Part model, mm, in its own coordinate system. Face numbers are marked on the shaded views. A direction names the side the tool comes from. Coordinates: 2 decimals unless noted, no trailing zeros. Write each loop counter-clockwise with the first axis right and the second up, starting at its lowest first coordinate (ties: lowest second). Pieces come first, ordered by that corner, then holes. Notation, with made-up numbers: (-2, -15.5) - (24, -15.5) arc R22 ccw to (24, -0.5) - close; hole circle Ø3 at (20.25, 32.25). An arc over 180 degrees is marked (long way). Use a Markdown table: item, result.
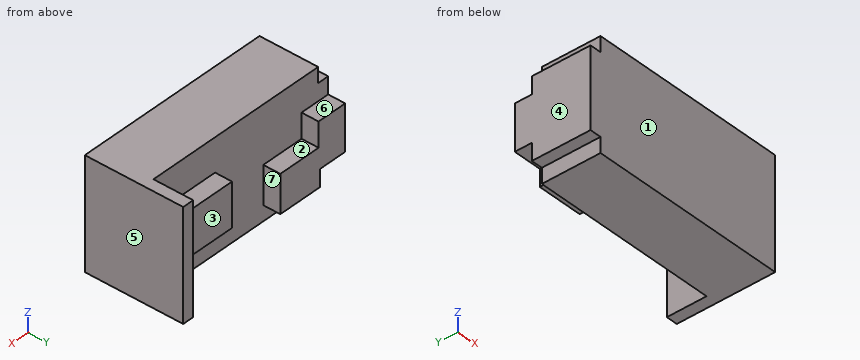
```python
from build123d import *

# Parameters (mm, degrees)
BOSS_EXTRUDE1_DEPTH = 29
SKETCH2_W           = 3
SKETCH2_H           = 4
CUT_EXTRUDE1_DEPTH  = 16.5
SKETCH3_W           = 18.5
SKETCH3_H           = 11.5
BOSS_EXTRUDE4_DEPTH = 4.5


with BuildPart() as part:
    # Sketch1 → Boss-Extrude1 (new body)
    with BuildSketch(Plane.XY):
        Polygon((0, 0), (0, 26), (-3, 26), (-3, 15.5), (-55.5, 15.5), (-55.5, 0), align=None)
    extrude(amount=BOSS_EXTRUDE1_DEPTH)

    # Sketch2 → Cut-Extrude1 (cut, through all)
    with BuildSketch(Plane(origin=(0, 15.5, 0), x_dir=(1, 0, 0), z_dir=(0, 1, 0))):
        with Locations((-54, -2)):
            Rectangle(SKETCH2_W, SKETCH2_H)
        with Locations((-54, -27)):
            Rectangle(SKETCH2_W, SKETCH2_H)
    extrude(amount=-CUT_EXTRUDE1_DEPTH, mode=Mode.SUBTRACT)

    # Sketch3 → Boss-Extrude4 (add)
    with BuildSketch(Plane(origin=(0, 15.5, 0), x_dir=(1, 0, 0), z_dir=(0, 1, 0))):
        with Locations((-12.25, -14.5)):
            Rectangle(SKETCH3_W, SKETCH3_H)
        Polygon((-55.5, -20.5), (-47.5, -20.5), (-47.5, -14), (-36, -14), (-36, -4), (-48, -4), (-48, -8.5), (-55.5, -8.5), align=None)
    extrude(amount=BOSS_EXTRUDE4_DEPTH)


solid = part.part
```
Item 1: Band-saw the part on C-C, the plane x = -41. Give the cut face in (y, z), then the cut area to 4 significant figures.
From the geometry:
| item | result |
|---|---|
| outline | (0, 0) - (15.5, 0) - (15.5, 4) - (20, 4) - (20, 14) - (15.5, 14) - (15.5, 29) - (0, 29) - close |
| area | 494.5 mm^2 |
Item 2: Two-plate mould, pull along X, no slides. Class the marked faces 4, 5, 6 and 7: pulls with the +X half, pulls with the -X half, needs draft (parallel to the pull), parting line crosses it, or undercut.
From the geometry:
| item | result |
|---|---|
| face 4 | pulls with the -X half |
| face 5 | pulls with the +X half |
| face 6 | needs draft |
| face 7 | undercut |
Item 3: Which spindle directions (+Z, -Z, +X, -X, +Y, -Y) get a long thin tool onto all of the face, cutting with end or side? Do the marked faces 1, 2 and 3. Say none if no direction does.
From the geometry:
| item | result |
|---|---|
| face 1 | +Z, -Z, +X, -X, -Y |
| face 2 | +Z, +Y |
| face 3 | +Z, -Z, -X, +Y |
Item 4: Band-saw the part on D-D, the plane z = 21.5. Give the cut face in (x, y).
From the geometry:
| item | result |
|---|---|
| outline | (-55.5, 0) - (0, 0) - (0, 26) - (-3, 26) - (-3, 15.5) - (-55.5, 15.5) - close |
Item 5: Drill centre lines: probe 1 along Y at (x, z) = (-49.5, 27.5); probe 2 along Z at (x, y) = (-8, 18); probe 3 along X at (y, z) = (5.5, 25.5). Where is each one in solid material? Low to high.
From the geometry:
| item | result |
|---|---|
| probe 1 | 0 to 15.5 |
| probe 2 | 8.75 to 20.25 |
| probe 3 | -52.5 to 0 |
Item 6: Band-saw the part on B-B, the plane z = 18.25. Give the cut face in (x, y), then the cut area to 3 significant figures.
From the geometry:
| item | result |
|---|---|
| outline | (-55.5, 0) - (0, 0) - (0, 26) - (-3, 26) - (-3, 20) - (-21.5, 20) - (-21.5, 15.5) - (-47.5, 15.5) - (-47.5, 20) - (-55.5, 20) - close |
| area | 1,010 mm^2 |
Item 7: Band-saw the part on A-A, the plane x = -13.5. Give the cut face in (y, z).
From the geometry:
| item | result |
|---|---|
| outline | (0, 0) - (15.5, 0) - (15.5, 8.75) - (20, 8.75) - (20, 20.25) - (15.5, 20.25) - (15.5, 29) - (0, 29) - close |
Item 8: Drop flat-ended pins along their axis: P1, Ø5, axis at y = 17.5, z = 17, coming from the +X side; P2, Ø3.5, axis at x = -50, y = 18.5, coming from the +Z side; P3, Ø2, axis at x = -13.5, y = 17, coming from the +Z side; P4, Ø14.5, axis at x = -20.5, z = 11.5, coming from the +Y side. Give the stop position or say it passes through.
From the geometry:
| item | result |
|---|---|
| P1 | x = 0 |
| P2 | z = 20.5 |
| P3 | z = 20.25 |
| P4 | y = 20 |
